```python
from build123d import *

# Parameters (mm, degrees)
SKETCH1_W                                        = 50.8
SKETCH1_H                                        = 50.8
BOSS_EXTRUDE1_DEPTH                              = 25.4
SKETCH7_W                                        = 50.8
SKETCH7_H                                        = 9.525
BOSS_EXTRUDE2_DEPTH                              = 19.05
SKETCH11_W                                       = 50.8
SKETCH11_H                                       = 9.525
BOSS_EXTRUDE3_DEPTH                              = 19.05
F_1_4_CLEARANCE_HOLE1_D                          = 6.7564
CBORE_FOR_1_4_SOCKET_HEAD_CAP_SCREW1_D           = 6.7564
CBORE_FOR_1_4_SOCKET_HEAD_CAP_SCREW1_CBORE_D     = 11.1125
CBORE_FOR_1_4_SOCKET_HEAD_CAP_SCREW1_CBORE_DEPTH = 6.35
LPATTERN1_COUNT                                  = 4
LPATTERN1_PITCH                                  = 25.4
LPATTERN1_COUNT_DIR2                             = 2
LPATTERN1_PITCH_DIR2                             = 25.4
LPATTERN2_COUNT                                  = 2
LPATTERN2_PITCH                                  = 25.4
LPATTERN2_COUNT_DIR2                             = 2
LPATTERN2_PITCH_DIR2                             = 25.4


with BuildPart() as part:
    # Sketch1 → Boss-Extrude1 (new body)
    with BuildSketch(Plane(origin=(0, 0, 0), x_dir=(1, 0, 0), z_dir=(0, 1, 0))):
        with Locations((25.4, 25.4)):
            Rectangle(SKETCH1_W, SKETCH1_H)
    extrude(amount=BOSS_EXTRUDE1_DEPTH)

    # Sketch7 → Boss-Extrude2 (add)
    with BuildSketch(Plane(origin=(0, 0, -50.8), x_dir=(-1, 0, 0), z_dir=(0, 0, -1))):
        with Locations((-25.4, 20.6375)):
            Rectangle(SKETCH7_W, SKETCH7_H)
    extrude(amount=BOSS_EXTRUDE2_DEPTH)

    # Sketch11 → Boss-Extrude3 (add)
    with BuildSketch(Plane.XY):
        with Locations((25.4, 20.6375)):
            Rectangle(SKETCH11_W, SKETCH11_H)
    extrude(amount=BOSS_EXTRUDE3_DEPTH)

    # 1/4 Clearance Hole1 (through all)
    with Locations(Plane(origin=(0, 25.4, 0), x_dir=(-1, 0, 0), z_dir=(0, 1, 0))):
        with Locations((-12.7, -63.5)):
            f_1_4_clearance_hole1 = Hole(F_1_4_CLEARANCE_HOLE1_D / 2)

    # CBORE for 1/4 Socket Head Cap Screw1 (through all)
    with Locations(Plane(origin=(0, 25.4, 0), x_dir=(-1, 0, 0), z_dir=(0, 1, 0))):
        with Locations((-12.7, -12.7)):
            cbore_for_1_4_socket_head_cap_screw1 = CounterBoreHole(CBORE_FOR_1_4_SOCKET_HEAD_CAP_SCREW1_D / 2, CBORE_FOR_1_4_SOCKET_HEAD_CAP_SCREW1_CBORE_D / 2, CBORE_FOR_1_4_SOCKET_HEAD_CAP_SCREW1_CBORE_DEPTH)

    # LPattern1: 1_4 Clearance Hole1 4 × 2
    with Locations(*[(j * LPATTERN1_PITCH_DIR2, 0, i * LPATTERN1_PITCH) for i in range(LPATTERN1_COUNT) for j in range(LPATTERN1_COUNT_DIR2) if (i, j) != (0, 0)]):
        add(f_1_4_clearance_hole1, mode=Mode.SUBTRACT)

    # LPattern2: CBORE for 1_4 Socket Head Cap Screw1 2 × 2
    with Locations(*[(j * LPATTERN2_PITCH_DIR2, 0, -i * LPATTERN2_PITCH) for i in range(LPATTERN2_COUNT) for j in range(LPATTERN2_COUNT_DIR2) if (i, j) != (0, 0)]):
        add(cbore_for_1_4_socket_head_cap_screw1, mode=Mode.SUBTRACT)


solid = part.part
```
CAD build for the part. Positions are in the model's coordinates, mm. A direction names the side the tool comes from. Coordinates: 2 decimals unless noted, no trailing zeros. Write each loop counter-clockwise with the first axis right and the second up, starting at its lowest first coordinate (ties: lowest second). Pieces come first, ordered by that corner, then holes.
(1) Flat gauge pins, fed straight in: pin 1 (6 mm diameter, centred on x = 37.5, z = -39, fed in from +Y); pin 2 (5.5 mm diameter, centred on x = 28, z = 6, fed in from -Y) (3 decimals); pin 3 (12.5 mm diameter, centred on x = 17, y = 6.5, fed in from -Z); pin 4 (4 mm diameter, centred on x = 12.7, z = -38.1, fed in from +Y). Where does each tip first touch, or does it go through?
(2) Cut at B-B, the plane z = -38.1. List the corners of the cut face in (x, y), and give its area (3 significant figures).
(3) Drill centre lines: probe 1 along Z at (x, y) = (12.7, 19); probe 2 along Z at (x, y) = (12.7, 20.75); probe 3 along X at (y, z) = (21.25, 15.5). Where is each one in solid material? Low to high.
(4) Cut at A-A, the plane x = 38.1. Count the separate pieces of the cut face and the enclosed holes in it, and give its area (3 significant figures).
(5) Cut at D-D, the plane y = 7.25. List the corners of the cut face in (x, z).
(6) Two-plate mould, pull along Z, no slides. Class faces 1 (the face through (41.221, 20.571, 11.406)), 2 (the face through (25, 21, 19.05)), 3 (the face through (26, 21, -69.85)): +Z half, -Z half, draft (parallel to the pull), parting line (faces both ways), or undercut.
(7) 3-axis set-ups, long thin cutter, end or side, ignore diameter. For faces 4 (the face through (25, 8, 0)), 5 (the face through (12.26, 9.39, -34.75)), 6 (the face through (38, 19.05, -42)): which of +Z, -Z, +X, -X, +Y, -Y reach the whole face in a straight line?
Geometry says:
1. pin 1: stops at y = 19.05
1. pin 2: stops at y = 15.875
1. pin 3: stops at z = -50.8
1. pin 4: passes through
2. outline: (0, 0) - (9.32, 0) - (9.32, 19.05) - (7.14, 19.05) - (7.14, 25.4) - (0, 25.4) - close; (16.08, 0) - (34.72, 0) - (34.72, 19.05) - (32.54, 19.05) - (32.54, 25.4) - (18.26, 25.4) - (18.26, 19.05) - (16.08, 19.05) - close; (41.48, 0) - (50.8, 0) - (50.8, 25.4) - (43.66, 25.4) - (43.66, 19.05) - (41.48, 19.05) - close
2. area: 892 mm2
3. probe 1: z = -69.85 to -66.88, -60.12 to -41.48, -34.72 to -16.08, -9.32 to 9.32, 16.08 to 19.05
3. probe 2: z = -69.85 to -66.88, -60.12 to -43.66, -32.54 to -18.26, -7.14 to 9.32, 16.08 to 19.05
3. probe 3: x = 0 to 10.81, 14.59 to 36.21, 39.99 to 50.8
4. separate pieces: 5
4. enclosed holes: 0
4. area: 1,130 mm2
5. outline: (0, -50.8) - (50.8, -50.8) - (50.8, 0) - (0, 0) - close; hole circle Ø6.76 at (12.7, -38.1); hole circle Ø6.76 at (12.7, -12.7); hole circle Ø6.76 at (38.1, -38.1); hole circle Ø6.76 at (38.1, -12.7)
6. face 1: undercut
6. face 2: +Z half
6. face 3: -Z half
7. face 4: +Z, +X, -X, -Y
7. face 5: +Y, -Y
7. face 6: +Y
